```python
from build123d import *

# Parameters (mm, degrees)
SKETCH1_R           = 2.9
SKETCH1_R_2         = 1.35
SKETCH1_R_3         = 1.6
BOSS_EXTRUDE1_DEPTH = 5
CUT_EXTRUDE1_DEPTH  = 5
CUT_EXTRUDE2_DEPTH  = 5
CHAMFER1_SIZE       = 0.4
CHAMFER2_SIZE       = 0.2
FILLET1_R           = 3
FILLET2_R           = 2
FILLET3_R           = 1
SKETCH4_W           = 20.9
SKETCH4_H           = 6.076557184
CUT_EXTRUDE3_DEPTH  = 1.7
SKETCH5_W           = 8
SKETCH5_H           = 9.98481564
CUT_EXTRUDE5_DEPTH  = 1.7
CUT_EXTRUDE6_DEPTH  = 1.7


with BuildPart() as part:
    # Sketch1 → Boss-Extrude1 (new body)
    with BuildSketch(Plane.XY):
        with BuildLine():
            Line((0, 0), (0, 83.4))
            ThreePointArc((0, 83.4), (1.464466094, 86.935533906), (5, 88.4))
            Line((5, 88.4), (49, 88.4))
            ThreePointArc((49, 88.4), (52.535533906, 86.935533906), (54, 83.4))
            Line((54, 83.4), (54, 0))
            Line((54, 0), (54, -32.8))
            Line((54, -32.8), (0, -32.8))
            Line((0, -32.8), (0, 0))
        make_face()
        with Locations((7, 83.4)):
            Circle(SKETCH1_R, mode=Mode.SUBTRACT)
        with Locations((47, 83.4)):
            Circle(SKETCH1_R, mode=Mode.SUBTRACT)
        with Locations((2.9, 54.7)):
            Circle(SKETCH1_R_2, mode=Mode.SUBTRACT)
        with Locations((51.1, 53.4)):
            Circle(SKETCH1_R_2, mode=Mode.SUBTRACT)
        with Locations((8, 2.6)):
            Circle(SKETCH1_R_2, mode=Mode.SUBTRACT)
        with Locations((35.9, 2.6)):
            Circle(SKETCH1_R_2, mode=Mode.SUBTRACT)
        with Locations((2.9, -27.8)):
            Circle(SKETCH1_R_3, mode=Mode.SUBTRACT)
        with Locations((51.1, -21.6)):
            Circle(SKETCH1_R_3, mode=Mode.SUBTRACT)
    extrude(amount=BOSS_EXTRUDE1_DEPTH)

    # Sketch2 → Cut-Extrude1 (cut)
    with BuildSketch(Plane.XY.offset(5)):
        Polygon((5.5, -32.8), (3, -30.3), (0, -30.3), (0, -32.8), align=None)
        Polygon((38.4, -32.8), (40.9, -30.3), (54, -30.3), (54, -32.8), align=None)
    extrude(amount=-CUT_EXTRUDE1_DEPTH, mode=Mode.SUBTRACT)

    # Sketch3 → Cut-Extrude2 (cut)
    with BuildSketch(Plane.XY.offset(5)):
        with BuildLine():
            Line((12, 81), (12, 78.4))
            Line((12, 78.4), (7.4, 78.4))
            ThreePointArc((7.4, 78.4), (3.864466094, 76.935533906), (2.4, 73.4))
            Line((2.4, 73.4), (2.4, 61.96963128))
            ThreePointArc((2.4, 61.96963128), (3.818077427, 58.48110284), (7.267932273, 56.971375773))
            Line((7.267932273, 56.971375773), (46.467932273, 55.935603416))
            ThreePointArc((46.467932273, 55.935603416), (50.088528441, 57.35193635), (51.6, 60.933858923))
            Line((51.6, 60.933858923), (51.6, 73.4))
            ThreePointArc((51.6, 73.4), (50.135533906, 76.935533906), (46.6, 78.4))
            Line((46.6, 78.4), (42, 78.4))
            Line((42, 78.4), (42, 81))
            ThreePointArc((42, 81), (40.535533906, 84.535533906), (37, 86))
            Line((37, 86), (17, 86))
            ThreePointArc((17, 86), (13.464466094, 84.535533906), (12, 81))
        make_face()
        with BuildLine():
            Line((7.532067727, 52.164396584), (46.732067727, 51.128624227))
            ThreePointArc((46.732067727, 51.128624227), (50.181922573, 49.61889716), (51.6, 46.13036872))
            Line((51.6, 46.13036872), (51.6, 10))
            ThreePointArc((51.6, 10), (50.135533906, 6.464466094), (46.6, 5))
            Line((46.6, 5), (7.4, 5))
            ThreePointArc((7.4, 5), (3.864466094, 6.464466094), (2.4, 10))
            Line((2.4, 10), (2.4, 47.166141077))
            ThreePointArc((2.4, 47.166141077), (3.911471559, 50.74806365), (7.532067727, 52.164396584))
        make_face()
        with BuildLine():
            Line((7.4, -1.076557184), (46.6, -1.076557184))
            ThreePointArc((46.6, -1.076557184), (50.135533906, -2.541023278), (51.6, -6.076557184))
            Line((51.6, -6.076557184), (51.6, -19.150510257))
            ThreePointArc((51.6, -19.150510257), (48.6, -21.6), (51.6, -24.049489743))
            Line((51.6, -24.049489743), (51.6, -24.9))
            ThreePointArc((51.6, -24.9), (50.721320344, -27.021320344), (48.6, -27.9))
            Line((48.6, -27.9), (6.148461174, -27.9))
            ThreePointArc((6.148461174, -27.9), (5.051673794, -25.364266048), (2.4, -24.588691855))
            Line((2.4, -24.588691855), (2.4, -6.076557184))
            ThreePointArc((2.4, -6.076557184), (3.864466094, -2.541023278), (7.4, -1.076557184))
        make_face()
    extrude(amount=-CUT_EXTRUDE2_DEPTH, mode=Mode.SUBTRACT)

    # Chamfer1
    chamfer1_edges = [part.edges().sort_by_distance(p)[0] for p in [
        (4.1, 83.4, 0),
        (4.1, 83.4, 5),
        (44.1, 83.4, 0),
        (44.1, 83.4, 5),
    ]]
    chamfer(chamfer1_edges, length=CHAMFER1_SIZE)

    # Chamfer2
    chamfer2_edges = [part.edges().sort_by_distance(p)[0] for p in [
        (1.55, 54.7, 0),
        (1.55, 54.7, 5),
        (49.75, 53.4, 0),
        (49.75, 53.4, 5),
        (6.65, 2.6, 0),
        (6.65, 2.6, 5),
        (34.55, 2.6, 0),
        (34.55, 2.6, 5),
    ]]
    chamfer(chamfer2_edges, length=CHAMFER2_SIZE)

    # Fillet1
    fillet1_edges = [part.edges().sort_by_distance(p)[0] for p in [
        (42, 78.4, 2.5),
        (12, 78.4, 2.5),
    ]]
    fillet(fillet1_edges, radius=FILLET1_R)

    # Fillet2
    fillet2_edges = [part.edges().sort_by_distance(p)[0] for p in [
        (0, -30.3, 2.5),
        (54, -30.3, 2.5),
    ]]
    fillet(fillet2_edges, radius=FILLET2_R)

    # Fillet3
    fillet3_edges = [part.edges().sort_by_distance(p)[0] for p in [
        (51.6, -24.049489743, 2.5),
        (51.6, -19.150510257, 2.5),
        (6.148461174, -27.9, 2.5),
        (2.4, -24.588691855, 2.5),
    ]]
    fillet(fillet3_edges, radius=FILLET3_R)

    # Sketch4 → Cut-Extrude3 (cut)
    with BuildSketch(Plane.XY.offset(5)):
        with Locations((21.95, 1.961721408)):
            Rectangle(SKETCH4_W, SKETCH4_H)
    extrude(amount=-CUT_EXTRUDE3_DEPTH, mode=Mode.SUBTRACT)

    # Sketch5 → Cut-Extrude5 (cut)
    with BuildSketch(Plane.XY.offset(5)):
        Polygon((2, 51.696310663), (52, 50.375172451), (52, -28.3), (2, -28.3), align=None)
        with Locations((6, 62.69240782)):
            Rectangle(SKETCH5_W, SKETCH5_H)
    extrude(amount=-CUT_EXTRUDE5_DEPTH, mode=Mode.SUBTRACT)

    # Sketch6 → Cut-Extrude6 (cut)
    with BuildSketch(Plane.XY.offset(5)):
        Polygon((48.1, 53.891781634), (5.9, 55.006822285), (5.9, 50.553811317), (48.1, 49.438770667), align=None)
    extrude(amount=-CUT_EXTRUDE6_DEPTH, mode=Mode.SUBTRACT)


solid = part.part
```
Can you work these out from the model? Positions are in its coordinate system, mm. A direction names the side the tool comes from. Round coordinates to 2 decimals unless told otherwise and drop trailing zeros. Order: outer loops, then holes, each group sorted by start corner. A loop starts at its lowest first (then second) coordinate and runs counter-clockwise, first axis right, second up.
(1) If we section it at B-B (x = 20.5): Please give me the cut outline in (y, z).
Results are:
outline: (-32.8, 0) - (-27.9, 0) - (-27.9, 3.3) - (-28.3, 3.3) - (-28.3, 5) - (-32.8, 5) - close; (-1.08, 0) - (5, 0) - (5, 3.3) - (-1.08, 3.3) - close; (51.82, 0) - (56.62, 0) - (56.62, 5) - (54.62, 5) - (54.62, 3.3) - (51.82, 3.3) - close; (86, 0) - (88.4, 0) - (88.4, 5) - (86, 5) - close
(2) If I drill on L1, parallel to X at y = 2.6, z = 2.25; L2, parallel to Y at x = 47, z = 2.4; L3, parallel to X at y = -21.6, z = 3.65, over which ranges is the centre line in solid material (lowest first)?
Results are:
L1: x = 0 to 6.65, 9.35 to 34.55, 37.25 to 54
L2: y = -30.3 to -27.9, -1.09 to 5.02, 51.11 to 55.95, 78.38 to 80.5, 86.3 to 88.4
L3: x = 0 to 2, 52.7 to 54
(3) If we section it at C-C (y = -14.5): Please give me the cut outline in (x, z).
Results are:
outline: (0, 0) - (2.4, 0) - (2.4, 3.3) - (2, 3.3) - (2, 5) - (0, 5) - close; (51.6, 0) - (54, 0) - (54, 5) - (52, 5) - (52, 3.3) - (51.6, 3.3) - close
(4) If we section it at A-A (y = 2.6): Please give me the cut outline in (x, z), plus the area to 3 significant figures.
Results are:
outline: (0, 0) - (6.45, 0) - (6.65, 0.2) - (6.65, 3.3) - (2, 3.3) - (2, 5) - (0, 5) - close; (9.35, 0.2) - (9.55, 0) - (34.35, 0) - (34.55, 0.2) - (34.55, 3.3) - (9.35, 3.3) - close; (37.25, 0.2) - (37.45, 0) - (54, 0) - (54, 5) - (52, 5) - (52, 3.3) - (37.25, 3.3) - close
area: 167 mm2
(5) If we section it at D-D (x = 35.9): Please give me the cut outline in (y, z), plus the area to 3 significant figures.
Results are:
outline: (-32.8, 0) - (-27.9, 0) - (-27.9, 3.3) - (-28.3, 3.3) - (-28.3, 5) - (-32.8, 5) - close; (-1.08, 0) - (1.05, 0) - (1.25, 0.2) - (1.25, 3.3) - (-1.08, 3.3) - close; (3.95, 0.2) - (4.15, 0) - (5, 0) - (5, 3.3) - (3.95, 3.3) - close; (51.41, 0) - (56.21, 0) - (56.21, 5) - (54.21, 5) - (54.21, 3.3) - (51.41, 3.3) - close; (86, 0) - (88.4, 0) - (88.4, 5) - (86, 5) - close
area: 66.2 mm2
(6) On a 3-axis mill with a long thin cutter (end or side, diameter ignored), from which of +Z, -Z, +X, -X, +Y, -Y can I reach the whole of each face in a straight line? I mean faces 1 (the face through (46, -30.3, 3)), 2 (the face through (1.43, 86.9, 2.46)), 3 (the face through (48.6, -21.5, 1.7)). Say none if no direction works.
Results are:
face 1: +Z, -Z, +X, -Y
face 2: +Z, -Z, -X, +Y
face 3: +Z, -Z
(7) We'd pull the mould along X, two halves only. Please class faces 4 (the face through (22, -32.8, 2)), 5 (the face through (3.9, 76.97, 2.54)), 6 (the face through (5.107, -25.414, 1.673)), 7 (the face through (4.3, -31.6, 2.5)): +X half, -X half, draft (parallel to the pull), parting line (faces both ways), or undercut.
Results are:
face 4: draft
face 5: undercut
face 6: undercut
face 7: -X half
(8) I'm going to push flat-ended pins straight in: pin 1 (1.5 mm diameter, centred on x = 44, z = 2.5, fed in from -Y); pin 2 (2.5 mm diameter, centred on x = 35.9, y = 2.6, fed in from +Z); pin 3 (2 mm diameter, centred on x = 27.5, y = 52, fed in from +Z); pin 4 (9.5 mm diameter, centred on x = 47, y = 83.4, fed in from -Z). Where does each tip first touch, or does it pass through?
Results are:
pin 1: stops at y = -30.3
pin 2: passes through
pin 3: stops at z = 3.3
pin 4: stops at z = 0
